Could you check a few things on this model? Use its own coordinates, in mm. Face numbers are marked on the shaded views. A direction names the side the tool comes from. Round coordinates to 2 decimals unless told otherwise and drop trailing zeros. Loops run counter-clockwise (first coordinate to the right, second up) from the corner with the lowest first, then second, coordinate; pieces in that order, holes last.
from build123d import *

# Parameters (mm, degrees)
F0_W          = 5.842
F0_H          = 12.7
F0_R          = 3.175
F2_DEPTH      = 3.175
F3_R          = 1.524
F4_DEPTH      = 1.27
F4_DEPTH_BACK = 6.35
F5_R          = 1.524
F6_DEPTH      = 10.414
F7_R          = 1.524
F8_DEPTH      = 17.78
F9_DEPTH      = 56.134


with BuildPart() as f1:
    # F0 (on Front) → F1 (revolve)
    with BuildSketch(Plane.XZ):
        Polygon((5.842, 12.7), (5.842, 0), (66.294, 0), (66.294, 12.7), (56.134, 12.7), (56.134, 10.16), (10.16, 10.16), (10.16, 12.7), align=None)
        with Locations((2.921, 6.35)):
            Rectangle(F0_W, F0_H)
    revolve(axis=Axis((33.147, 0, 0), (-1, 0, 0)))

    # F0 (on Front) → F2 (join, symmetric)
    with BuildSketch(Plane.XZ):
        with Locations((2.921, 6.35)):
            Rectangle(F0_W, F0_H)
        with BuildLine():
            Line((-0.9398, 0), (0, 0))
            Line((0, 0), (0, 12.7))
            Line((0, 12.7), (5.842, 12.7))
            Line((5.842, 12.7), (5.842, 15.24))
            Line((5.842, 15.24), (-0.508, 15.24))
            Line((-0.508, 15.24), (-10.8806298187, 3.8475430269))
            ThreePointArc((-10.8806298187, 3.8475430269), (-4.5919612295, 5.3297205562), (-0.9398, 0))
        make_face()
        with BuildLine():
            ThreePointArc((-8.1826630726, -5.5069827884), (-3.1957909266, -4.5493385486), (-0.9398, 0))
            ThreePointArc((-0.9398, 0), (-4.5919612295, 5.3297205562), (-10.8806298187, 3.8475430269))
            ThreePointArc((-10.8806298187, 3.8475430269), (-12.1459778134, -1.5837270034), (-8.1826630726, -5.5069827884))
        make_face()
        with Locations((-6.6548, 0)):
            Circle(F0_R, mode=Mode.SUBTRACT)
        with BuildLine():
            Line((5.842, 0), (0, 0))
            Line((0, 0), (-0.9398, 0))
            ThreePointArc((-0.9398, 0), (-3.1957909266, -4.5493385486), (-8.1826630726, -5.5069827884))
            Line((-8.1826630726, -5.5069827884), (5.842, -9.398))
            Line((5.842, -9.398), (5.842, 0))
        make_face()
    extrude(amount=F2_DEPTH, both=True)

    # F3 (on face) → F4 (join, two sides)
    with BuildSketch(Plane.YZ.offset(66.294)) as f4_sk:
        with BuildLine():
            ThreePointArc((-5.08, 0), (0, -5.08), (5.08, 0))
            ThreePointArc((5.08, 0), (0, 5.08), (-5.08, 0))
        make_face()
        Circle(F3_R, mode=Mode.SUBTRACT)
        with BuildLine():
            ThreePointArc((-5.08, 0), (0, 5.08), (5.08, 0))
            Line((5.08, 0), (5.08, 15.24))
            Line((5.08, 15.24), (-5.08, 15.24))
            Line((-5.08, 15.24), (-5.08, 0))
        make_face()
    extrude(amount=-F4_DEPTH)
    extrude(f4_sk.sketch, amount=F4_DEPTH_BACK)

    # F5 (on face) → F6 (cut)
    with BuildSketch(Plane.XY.offset(15.24)):
        with Locations((68.834, 0)):
            Circle(F5_R)
    extrude(amount=-F6_DEPTH, mode=Mode.SUBTRACT)

    # F7 (on face) → F8 (cut)
    with BuildSketch(Plane.XY.offset(15.24)):
        with Locations((2.667, 0)):
            Circle(F7_R)
    extrude(amount=-F8_DEPTH, mode=Mode.SUBTRACT)

    # F9 (add, through all): a face of the model
    f9_faces = [f1.faces().sort_by_distance(p)[0] for p in [
        (66.294, 0, 0),
    ]]
    extrude(f9_faces, amount=-F9_DEPTH)


solid = f1.part
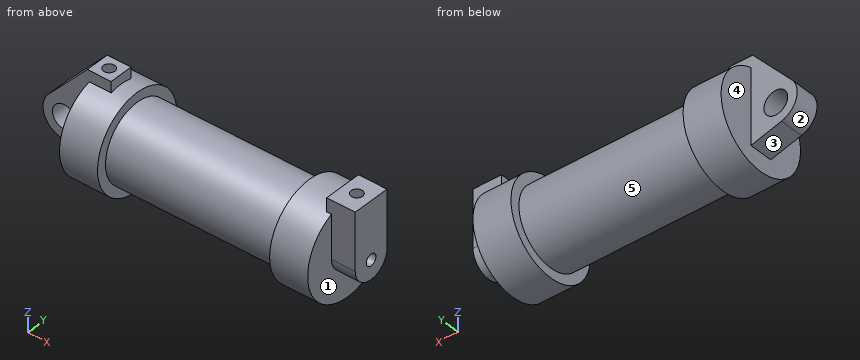
Item 1: If I drill on line 1 along X through (y, z) = (7, -8.5); line 2 along Z through (x, y) = (69, 0); line 3 along X through (y, z) = (4.5, 0.5), over which ranges is the centre line in solid material (lowest first)?
Results list:
line 1: x = 0 to 10.16, 56.13 to 66.29
line 2: z = -5.08 to -1.52, 1.52 to 4.83
line 3: x = 0 to 72.64
Item 2: If we section it at B-B, the plane z = -0.75: Count the separate pieces of the cut face and the enclosed holes in it, then the cut area to 3 significant figures.
Results list:
separate pieces: 2
enclosed holes: 1
area: 1,530 mm2
Item 3: If we section it at D-D, the plane x = 12: Please give me the cut outline in (y, z).
Results list:
outline: circle Ø20.32 at (0, 0)
Item 4: Will these pins go through, and if not, where does the flat tip stop? pin 1 (2 mm diameter, centred on x = 10.5, z = 3.5, fed in from +Y); pin 2 (2 mm diameter, centred on x = 16.5, y = -8, fed in from +Z); pin 3 (7.5 mm diameter, centred on y = -4.5, z = -6, fed in from -X).
Results list:
pin 1: stops at y = 12.44
pin 2: stops at z = 7.36
pin 3: stops at x = -11.8
Item 5: If we section it at C-C, the plane y = 8.25: Please give me the cut outline in (x, z).
Results list:
outline: (0, -9.66) - (10.16, -9.66) - (10.16, -5.93) - (56.13, -5.93) - (56.13, -9.66) - (66.29, -9.66) - (66.29, 9.66) - (56.13, 9.66) - (56.13, 5.93) - (10.16, 5.93) - (10.16, 9.66) - (0, 9.66) - close
Item 6: For the marked faces 1, 2, 3, 4 and 5, which set-ups out of +Z, -Z, +X, -X, +Y, -Y let a thin tool reach every point of the face, with its end or its side?
Results list:
face 1: -Z, +X
face 2: -X, +Y, -Y
face 3: -Z, -X, +Y, -Y
face 4: -Z, -X
face 5: none
